Autodesk Inventor part; units mm, degrees
ref_plane "YZ Plane" through (0, 0, 0) normal (1, 0, 0) x (0, 1, 0)
ref_plane "XZ Plane" through (0, 0, 0) normal (0, 1, 0) x (-1, 0, 0)
ref_plane "XY Plane" through (0, 0, 0) normal (0, 0, 1) x (1, 0, 0)
sketch "Sketch1" plane through (0, 0, 0) normal (0, 0, 1) x (1, 0, 0)
  line L0 (0, 0) -> (-100, 0)
  line L1 (-100, 0) -> (-100, 33) construction
  line L2 (-100, 33) -> (0, 36)
  line L3 (0, 36) -> (0, 0)
  arc A0 (-160, 20) -> (-100, 0) centre (-100, 100) ccw
  arc A1 (-100, 33) -> (-160, 20) centre (-94.9522, -135.2589) ccw
  dimension "d0" = 100
  dimension "d2" = 36
  dimension "d10" = 60
  dimension "d11" = 20
  dimension "d12" = 33
extrude "Extrusion1" add sketch "Sketch1" along normal mid plane 1.1
sketch "Sketch2" plane through (0, 0, 0) normal (0, 0, 1) x (1, 0, 0)
  line L0 (0, 36) -> (-160.3357, 31.1899)
  line L1 (0, 36) -> (86.8358, 36)
  line L2 (86.8358, 36) -> (86.8358, 12.7298)
  line L3 (86.8358, 12.7298) -> (0, 12.7298)
  line L4 (0, 12.7298) -> (0, 36)
  point P0 (0, 0)
  point P1 (-160, 20)
extrude "Extrusion2" add sketch "Sketch2" along normal mid plane 15
chamfer "Chamfer1" distance 0.5 angle 45 4 edges at (-50, 0, 0.55) (-131.6228, 5.1317, 0.55) (-50, 0, -0.55) (-131.6228, 5.1317, -0.55)
properties part number "Knife"
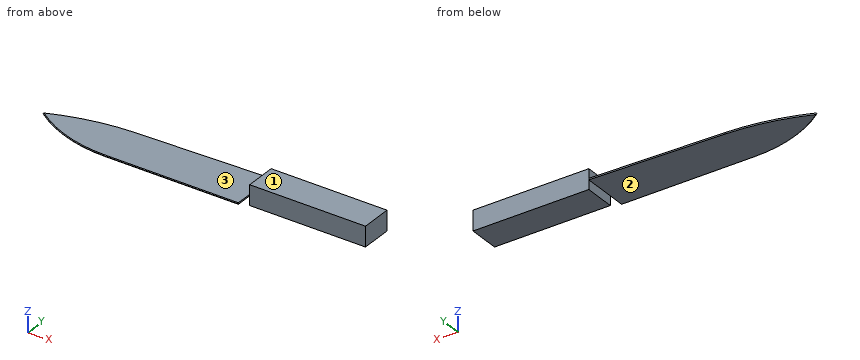
Check sheet for the modelled part. Datum: model origin and axes. Units: mm. Face numbers are marked on the shaded views. A direction names the side the tool comes from. Give positions to 0.01 mm unless a question says otherwise; leave off trailing zeros. Write each loop counter-clockwise with the first axis right and the second up, starting at its lowest first coordinate (ties: lowest second). Pieces come first, ordered by that corner, then holes. Notation, with made-up numbers: M -0.5,55.25 L 49.5,55.25 A19 ccw 49.5,61.25 Z; hole C -23,58 d7. An arc over 180 degrees is marked long. Use one line per item in the form item = value.
(1) Section check B-B on y = 23.5. Record the boundary of the cut face in (x, z), plus the area to 3 significant figures.
Answer block:
outline = M -150.92,-0.55 L 0,-0.55 L 0,-7.5 L 86.84,-7.5 L 86.84,7.5 L 0,7.5 L 0,0.55 L -150.92,0.55 Z
area = 1,470 mm2
(2) Section check C-C on z = 4. Record the boundary of the cut face in (x, y), plus the area to 3 significant figures.
Answer block:
outline = M 0,12.73 L 86.84,12.73 L 86.84,36 L 0,36 Z
area = 2,020 mm2
(3) Material ranges on line 1 along X through (y, z) = (14, 5); line 2 along Z through (x, y) = (-90, 20); line 3 along Y through (x, z) = (72, -0.5), recorded low to high.
Answer block:
line_1 = 0 to 86.84
line_2 = -0.55 to 0.55
line_3 = 12.73 to 36
(4) Tool access check on the marked faces 1, 2 and 3. Record the directions out of +Z, -Z, +X, -X, +Y, -Y that give a thin tool (end or side, any length) a straight path to the whole face; none if there is none.
Answer block:
face_1 = +Z, +X, -X, +Y, -Y
face_2 = -Z, -X, +Y, -Y
face_3 = +Z, -X, +Y, -Y
(5) Section check A-A on x = -75. Record the boundary of the cut face in (y, z), plus the area to 3 significant figures.
Answer block:
outline = M 0,-0.05 L 0.5,-0.55 L 33.75,-0.55 L 33.75,0.55 L 0.5,0.55 L 0,0.05 Z
area = 36.9 mm2
(6) Depth check by flat-ended pin: P1, Ø8, axis at x = -21, y = 4, coming from the +Z side; P2, Ø0.6, axis at y = 8.5, z = 0, coming from the +X side; P3, Ø6, axis at y = 7.5, z = -4, coming from the -X side; P4, Ø3.5, axis at y = 29, z = 3, coming from the -X side. Enter the tip coordinate at first touch or a pass-through.
Answer block:
P1 = 0.55
P2 = 0
P3 = through
P4 = 0
(7) Section check D-D on x = 13.5. Record the boundary of the cut face in (y, z), plus the area to 3 significant figures.
Answer block:
outline = M 12.73,-7.5 L 36,-7.5 L 36,7.5 L 12.73,7.5 Z
area = 349 mm2
